Source: CAD feature listing. Evaluate the final solid. Frame: model axes, mm. A direction names the side the tool comes from. Coordinates: 2 decimals unless noted, no trailing zeros. Order: outer loops, then holes, each group sorted by start corner. A loop starts at its lowest first (then second) coordinate and runs counter-clockwise, first axis right, second up.
Item 1: Section D-D on z = 8.5. Return the cut outline in (x, y).
Item 2: Section C-C on z = -4.5. Return the cut outline in (x, y).
Item 3: Mould query, pull axis Z, two halves, no side actions, for faces 1 (the flat face through (0.11, 7.02, -26.71)), 2 (the flat face through (-7.938, 8, -11)), 3 (the flat face through (10.312, 13, 18)). Classes: released by +Z, released by -Z, zero draft, split by the parting line, or undercut.
Item 4: Ray query, line 1 (X direction, y = 8.75, z = 16); line 2 (Z direction, x = 6.5, y = 10); line 3 (Y direction, x = 6.75, z = -14.5). Return the intervals inside material, ascending.
Item 5: Section B-B on y = 10.5. Return the cut outline in (x, z).
Item 6: Contact query for flat-ended pins moving along their axis: P1, Ø1, axis at y = 7.5, z = -13.5, coming from the -X side; P2, Ø6, axis at x = 7, z = 23, coming from the +Y side; P3, Ø3, axis at y = 6.5, z = 21.5, coming from the -X side; P4, Ø1.5, axis at x = -1, z = 14, coming from the +Y side. Output: stop coordinate, or through.
Item 7: Section A-A on x = 3.5. Return the cut outline in (y, z) (3 decimals).
Item 8: Reachability of faces 4 (the flat face through (0.111, 2.114, 13.52)), 5 (the flat face through (0, 14, 7.823)), 6 (the flat face through (0, 12.495, -39)) from +Z, -Z, +X, -X, +Y, -Y: full face, straight path, thin tool, end or side. Return the list, or none.
from build123d import *

# Parameters (mm, degrees)
BOSS_EXTRUDE1_DEPTH = 7.9375
BOSS_EXTRUDE2_DEPTH = 10.3124


with BuildPart() as part:
    # Sketch3 → Boss-Extrude1 (new, symmetric)
    with BuildSketch(Plane(origin=(0, 0, 0), x_dir=(0, 0, -1), z_dir=(1, 0, 0))):
        with BuildLine():
            Line((40.513, 14.235338715), (40.513, 12.495229879))
            Line((40.513, 12.495229879), (37.766212018, 12.495229879))
            Line((37.766212018, 12.495229879), (15.349467418, 1.395404479))
            Line((15.349467418, 1.395404479), (-10.837881782, 1.395404479))
            Line((-10.837881782, 1.395404479), (-16.27838917, 2.853173638))
            ThreePointArc((-16.27838917, 2.853173638), (-19.721025133, 8.005427537), (-15.0622, 12.0911112))
            Line((-15.0622, 12.0911112), (-9.601272901, 12.0911112))
            Line((-9.601272901, 12.0911112), (-7.8233016, 12.835531808))
            Line((-7.8233016, 12.835531808), (-7.8233016, 14.235338715))
            Line((-7.8233016, 14.235338715), (40.513, 14.235338715))
        make_face()
    extrude(amount=BOSS_EXTRUDE1_DEPTH, both=True)

    # Sketch4 → Boss-Extrude2 (add, symmetric)
    with BuildSketch(Plane(origin=(0, 0, 0), x_dir=(0, 0, -1), z_dir=(1, 0, 0))):
        with BuildLine():
            ThreePointArc((-3.239093433, 3.82959498), (-1.848605226, 3.466296321), (-1.485306567, 4.856784528))
            ThreePointArc((-1.485306567, 4.856784528), (-18.623790881, 14.266172543), (-35.024465128, 3.622765587))
            ThreePointArc((-35.024465128, 3.622765587), (-34.559965587, 2.262734872), (-33.199934872, 2.727234413))
            ThreePointArc((-33.199934872, 2.727234413), (-18.549060441, 12.235088571), (-3.239093433, 3.82959498))
        make_face()
    extrude(amount=BOSS_EXTRUDE2_DEPTH, both=True)


solid = part.part
Answer list:
1. outline: (-10.31, 9.4) - (-7.94, 9.4) - (-7.94, 1.4) - (7.94, 1.4) - (7.94, 9.4) - (10.31, 9.4) - (10.31, 11.79) - (7.94, 11.79) - (7.94, 12.55) - (-7.94, 12.55) - (-7.94, 11.79) - (-10.31, 11.79) - close
2. outline: (-7.94, 1.4) - (7.94, 1.4) - (7.94, 14.24) - (-7.94, 14.24) - close
3. face 1: released by -Z
3. face 2: undercut
3. face 3: zero draft
4. line 1: x = -7.94 to 7.94
4. line 2: z = -32.73 to 18.97, 26.37 to 29.95
4. line 3: y = 1.4 to 14.24
5. outline: (-10.31, 6.53) - (-7.94, 6.53) - (-7.94, -33.74) - (7.94, -33.74) - (7.94, 6.53) - (10.31, 6.53) - (10.31, 10.41) - (7.94, 10.41) - (7.94, 18.59) - (-7.94, 18.59) - (-7.94, 10.41) - (-10.31, 10.41) - close; (-10.31, 25.43) - (10.31, 25.43) - (10.31, 29.31) - (-10.31, 29.31) - close
6. P1: stops at x = -7.94
6. P2: stops at y = 14.17
6. P3: passes through
6. P4: stops at y = 14.01
7. outline: (1.395, -15.349) - (12.495, -37.766) - (12.495, -40.513) - (14.235, -40.513) - (14.235, 7.823) - (12.836, 7.823) - (12.216, 9.302) arc R19.05 ccw to (3.623, 35.024) arc R1.016 ccw to (2.727, 33.2) arc R17.018 cw to (12.072, 15.489) arc R4.699 ccw to (2.853, 16.278) - (1.395, 10.838) - close
8. face 4: +X, -X, -Y
8. face 5: +X, -X, +Y
8. face 6: -Z, +X, -X, -Y
